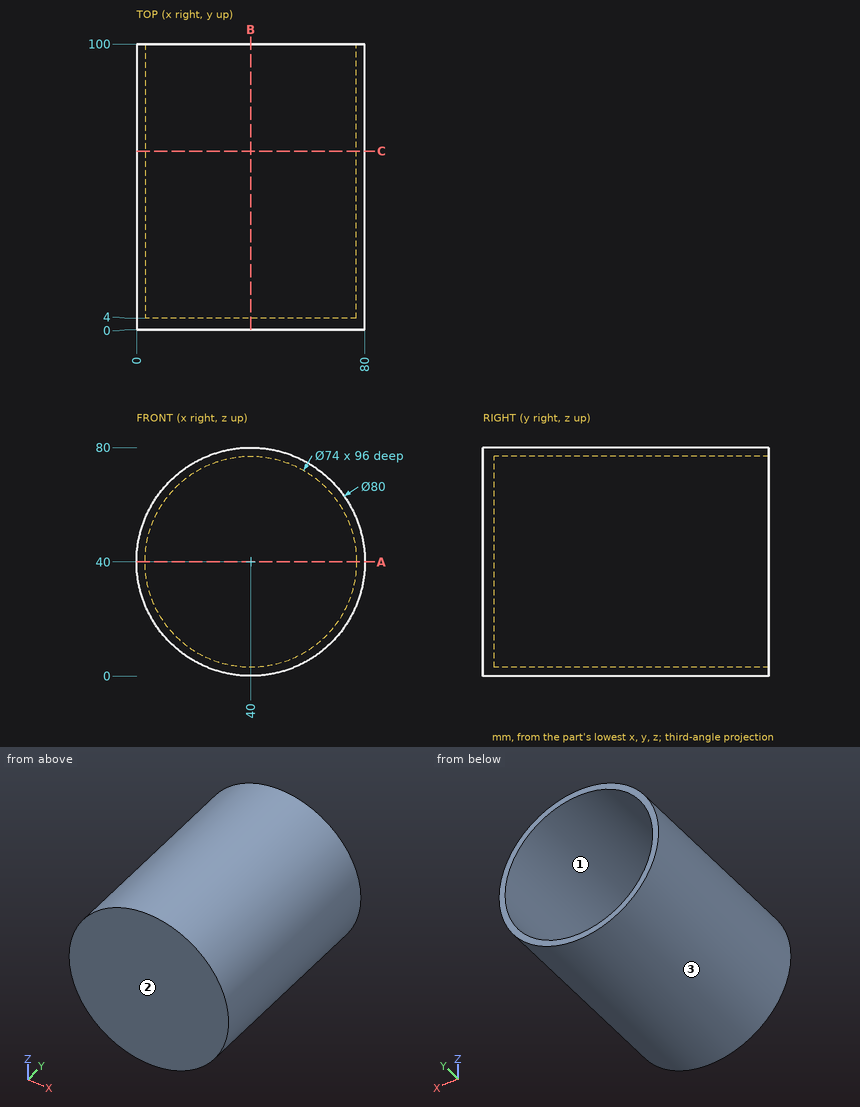
Input: dimensioned drawing with shaded views. Units: mm. Origin: part minimum x, y, z. Coordinates: 2 decimals unless noted, no trailing zeros. Order: outer loops, then holes, each group sorted by start corner. A loop starts at its lowest first (then second) coordinate and runs counter-clockwise, first axis right, second up. Notation, with made-up numbers: (14, -9.75) -> (57, -9.75) arc R15 ccw to (57, 18.25) -> close; hole circle Ø6 at (37, 25). An arc over 180 degrees is marked (long way). Use CSV: the item, a comma, the result in double quotes.
1) Line query: line 1 (Z direction, x = 40, y = 37.5); line 2 (Y direction, x = 32, z = 56). Output: solid intervals per line, ascending.
Findings:
line 1,"z = 0 to 3, 77 to 80"
line 2,"y = 0 to 4"
2) Pin query (flat end, axial travel): pin 1 Ø6 at (x, z) = (42.5, 55) entering from +Y; pin 2 Ø4 at (x, y) = (10.5, 78) entering from -Z; pin 3 Ø3 at (x, y) = (60, 25.5) entering from +Z. Return the tip coordinate at first contact, or that it passes through.
Findings:
pin 1,"stops at y = 4"
pin 2,"stops at z = 10.95"
pin 3,"stops at z = 75.46"
3) Mould query, pull axis Z, two halves, no side actions, for the marked faces 1, 2 and 3. Classes: +Z half, -Z half, draft (parallel to the pull), parting line (faces both ways), or undercut.
Findings:
face 1,"undercut"
face 2,"draft"
face 3,"parting line"
4) Section B-B on x = 40. Output: boundary loops of the cut face in (y, z).
Findings:
outline,"(0, 0) -> (100, 0) -> (100, 3) -> (4, 3) -> (4, 77) -> (100, 77) -> (100, 80) -> (0, 80) -> close"
5) Section A-A on z = 40. Output: boundary loops of the cut face in (x, y).
Findings:
outline,"(0, 0) -> (80, 0) -> (80, 100) -> (77, 100) -> (77, 4) -> (3, 4) -> (3, 100) -> (0, 100) -> close"
6) Section C-C on y = 62.5. Output: boundary loops of the cut face in (x, z), then the cut area to 3 significant figures.
Findings:
outline,"circle Ø80 at (40, 40); hole circle Ø74 at (40, 40)"
area,"726 mm^2"
